```python
from build123d import *

# Parameters (mm, degrees)
SKETCH_1_R          = 12
SKETCH_1_R_2        = 1.5
SKETCH_1_R_3        = 6.3
EXTRUDE_1_DEPTH     = 4
SKETCH_6_W          = 40
SKETCH_6_H          = 10
SKETCH_6_R          = 2
SKETCH_6_R_2        = 1.5
EXTRUDE_5_DEPTH     = 4
FILLET_1_R          = 10
FILLET_2_R          = 2
SKETCH_7_R          = 6.3
CUT_EXTRUDE_1_DEPTH = 5


with BuildPart() as part:
    # 草图1 → 凸台-拉伸1 (new body)
    with BuildSketch(Plane(origin=(0, 0, 0), x_dir=(0, 0, -1), z_dir=(1, 0, 0))):
        Circle(SKETCH_1_R)
        with Locations((0, 9)):
            Circle(SKETCH_1_R_2, mode=Mode.SUBTRACT)
        Circle(SKETCH_1_R_3, mode=Mode.SUBTRACT)
        with Locations((9, 0)):
            Circle(SKETCH_1_R_2, mode=Mode.SUBTRACT)
        with Locations((0, -9)):
            Circle(SKETCH_1_R_2, mode=Mode.SUBTRACT)
        with Locations((-9, 0)):
            Circle(SKETCH_1_R_2, mode=Mode.SUBTRACT)
    extrude(amount=EXTRUDE_1_DEPTH)

    # 草图6 → 凸台-拉伸5 (add)
    with BuildSketch(Plane(origin=(4, 0, 0), x_dir=(0, 0, -1), z_dir=(1, 0, 0))):
        with Locations((-25, 0)):
            Rectangle(SKETCH_6_W, SKETCH_6_H)
        with Locations((-40, 0)):
            Circle(SKETCH_6_R, mode=Mode.SUBTRACT)
        with Locations((-9, 0)):
            Circle(SKETCH_6_R_2, mode=Mode.SUBTRACT)
    extrude(amount=-EXTRUDE_5_DEPTH)

    # 圆角1
    fillet_1_edges = [part.edges().sort_by_distance(p)[0] for p in [
        (2, 5, 10.908712115),
        (2, -5, 10.908712115),
    ]]
    fillet(fillet_1_edges, radius=FILLET_1_R)

    # 圆角2
    fillet_2_edges = [part.edges().sort_by_distance(p)[0] for p in [
        (2, 5, 45),
        (2, -5, 45),
    ]]
    fillet(fillet_2_edges, radius=FILLET_2_R)

    # 草图7 → 切除-拉伸1 (cut, symmetric)
    with BuildSketch(Plane(origin=(4, 0, 0), x_dir=(0, 0, -1), z_dir=(1, 0, 0))):
        Circle(SKETCH_7_R)
    extrude(amount=CUT_EXTRUDE_1_DEPTH, both=True, mode=Mode.SUBTRACT)


solid = part.part
```
Can you work these out from the model? Positions are in its coordinate system, mm. A direction names the side the tool comes from. Round coordinates to 2 decimals unless told otherwise and drop trailing zeros. Order: outer loops, then holes, each group sorted by start corner. A loop starts at its lowest first (then second) coordinate and runs counter-clockwise, first axis right, second up.
(1) If we section it at A-A (z = 40): Please give me the cut outline in (x, y).
Results are:
outline: (0, -5) - (4, -5) - (4, -2) - (0, -2) - close; (0, 2) - (4, 2) - (4, 5) - (0, 5) - close
(2) If we section it at D-D (x = 1.1): Please give me the cut outline in (y, z).
Results are:
outline: (-8.18, 8.78) arc R12 ccw (long way) to (8.18, 8.78) arc R10 cw to (5, 16.09) - (5, 43) arc R2 ccw to (3, 45) - (-3, 45) arc R2 ccw to (-5, 43) - (-5, 16.09) arc R10 cw to start; hole circle Ø3 at (-9, 0); hole circle Ø12.6 at (0, 0); hole circle Ø4 at (0, 40); hole circle Ø3 at (0, -9); hole circle Ø3 at (0, 9); hole circle Ø3 at (9, 0)
(3) On a 3-axis mill with a long thin cutter (end or side, diameter ignored), from which of +Z, -Z, +X, -X, +Y, -Y can I reach the whole of each face in a straight line? I mean faces 5 (the face through (1.972, -5.853, 12.052)), 6 (the face through (2, 5, 30)). Say none if no direction works.
Results are:
face 5: +Z, +X, -X, -Y
face 6: +Z, +X, -X, +Y
(4) If I drill on L1, parallel to Y at x = 2.85, z = 0; L2, parallel to Y at x = 1.1, z = 40; L3, parallel to Z at x = 3.65, y = 1.25, over which ranges is the centre line in solid material (lowest first)?
Results are:
L1: y = -12 to -10.5, -7.5 to -6.3, 6.3 to 7.5, 10.5 to 12
L2: y = -5 to -2, 2 to 5
L3: z = -11.93 to -9.83, -8.17 to -6.17, 6.17 to 8.17, 9.83 to 38.44, 41.56 to 45
(5) If we section it at B-B (y = 0): Please give me the cut outline in (x, z), plus the area to 3 significant figures.
Results are:
outline: (0, -12) - (4, -12) - (4, -10.5) - (0, -10.5) - close; (0, -7.5) - (4, -7.5) - (4, -6.3) - (0, -6.3) - close; (0, 6.3) - (4, 6.3) - (4, 7.5) - (0, 7.5) - close; (0, 10.5) - (4, 10.5) - (4, 38) - (0, 38) - close; (0, 42) - (4, 42) - (4, 45) - (0, 45) - close
area: 138 mm2
(6) We'd pull the mould along Z, two halves only. Please class faces 1 (the face through (1.972, 5.853, 12.052)), 2 (the face through (2, -0.9, -7.8)), 3 (the face through (2, -5, 30)), 4 (the face through (2, 0, -12)): +Z half, -Z half, draft (parallel to the pull), parting line (faces both ways), or undercut.
Results are:
face 1: +Z half
face 2: undercut
face 3: draft
face 4: parting line
(7) I'm going to push flat-ended pins straight in: pin 1 (2 mm diameter, centred on x = 2.5, z = -4.5, fed in from -Y); pin 2 (1.5 mm diameter, centred on x = 0.5, y = -4.5, fed in from +Z); pin 3 (1 mm diameter, centred on x = 2.5, z = 33, fed in from +Y). Where does each tip first touch, or does it pass through?
Results are:
pin 1: stops at y = -11.48
pin 2: stops at z = 44.85
pin 3: stops at y = 5
(8) If we section it at C-C (y = -9): Please give me the cut outline in (x, z), plus the area to 3 significant figures.
Results are:
outline: (0, -7.94) - (4, -7.94) - (4, -1.5) - (0, -1.5) - close; (0, 1.5) - (4, 1.5) - (4, 7.94) - (0, 7.94) - close
area: 51.5 mm2
